For this review, take the finished solid that the model builds, in its own axes (mm). A direction names the side the tool comes from. Give positions to 0.01 mm unless a question says otherwise; leave off trailing zeros. Write each loop counter-clockwise with the first axis right and the second up, starting at its lowest first coordinate (ties: lowest second). Pieces come first, ordered by that corner, then holes. Notation, with made-up numbers: M -12,65.5 L 23,65.5 A23 ccw 23,75.5 Z; hole C 41,-16 d1. An arc over 180 degrees is marked long. Answer as a JSON object with one key per item and string values. Group by question number.
```python
from build123d import *

# Parameters (mm, degrees)
SKETCH_1_R           = 6
EXTRUDE_1_DEPTH      = 6
SKETCH_2_R           = 3
EXTRUDE_2_DEPTH      = 15
SKETCH_4_OUTSIDE_W   = 19.4
SKETCH_4_OUTSIDE_H   = 19.4
CUT_EXTRUDE_1_DEPTH  = 12
SKETCH_5_R           = 18.5
EXTRUDE_3_DEPTH      = 39
EXTRUDE_START        = 6
SKETCH_6_R           = 6
EXTRUDE_4_DEPTH      = 6
SKETCH_7_W           = 38
SKETCH_7_H           = 38
EXTRUDE_5_DEPTH      = 8
EXTRUDE_6_REACH      = 71.176
EXTRUDE_6_END_RADIUS = 18.5
SKETCH_8_W           = 38
SKETCH_8_H           = 26.2
SKETCH_9_R           = 17.9
EXTRUDE_7_DEPTH      = 27
SKETCH_10_R          = 5
EXTRUDE_8_DEPTH      = 2.5
SKETCH_11_R          = 1.5
CUT_EXTRUDE_2_DEPTH  = 4
FILLET_1_R           = 1.5


with BuildPart() as part:
    # Sketch 1 → Extrude 1 (new body)
    with BuildSketch(Plane.XY):
        Circle(SKETCH_1_R)
    extrude(amount=EXTRUDE_1_DEPTH)

    # Sketch 2 → Extrude 2 (add)
    with BuildSketch(Plane.XY.offset(6)):
        Circle(SKETCH_2_R)
    extrude(amount=EXTRUDE_2_DEPTH)

    # Sketch 4 outside → Cut-Extrude 1 (cut)
    with BuildSketch(Plane.XY.offset(21)):
        Rectangle(SKETCH_4_OUTSIDE_W, SKETCH_4_OUTSIDE_H)
        with BuildLine():
            Line((-1.658312395, 2.5), (1.658312395, 2.5))
            ThreePointArc((1.658312395, 2.5), (0, -3), (-1.658312395, 2.5))
        make_face(mode=Mode.SUBTRACT)
    extrude(amount=-CUT_EXTRUDE_1_DEPTH, mode=Mode.SUBTRACT)

    # Sketch 5 → Extrude 3 (add)
    with BuildSketch(Plane.XY):
        with Locations((0, -7)):
            Circle(SKETCH_5_R)
    extrude(amount=-EXTRUDE_3_DEPTH)

    # Sketch 6 → Extrude 4 (add)
    with BuildSketch(Plane(origin=(0, 0, -39), x_dir=(-1, 0, 0), z_dir=(0, 0, -1)).offset(EXTRUDE_START)):
        with Locations(Location((0, 0, 0), (0, 0, 180))):
            Circle(SKETCH_6_R)
    extrude(amount=-EXTRUDE_4_DEPTH)



with BuildPart() as body_2:
    # Sketch 7 → Extrude 5 (new body)
    with BuildSketch(Plane(origin=(26.5, 0, 0), x_dir=(0, 0, -1), z_dir=(1, 0, 0))):
        with Locations((19.5, -18.3)):
            Rectangle(SKETCH_7_W, SKETCH_7_H)
    extrude(amount=-EXTRUDE_5_DEPTH)


with BuildPart() as part_1:
    add(part.part)

    add(body_2.part)  # Extrude 6 merges body 2
    # Extrude 6: up to this cylinder (the profile starts outside it)
    extrude_6_end = Plane(origin=(0, -7, -19.5), z_dir=(0, 0, 1)) * Cylinder(EXTRUDE_6_END_RADIUS, 180.352, mode=Mode.PRIVATE)
    # Sketch 8 → Extrude 6 (add, up to the surface)
    with BuildSketch(Plane.ZY.offset(-18.5), mode=Mode.PRIVATE) as extrude_6_sk1:
        with Locations((-19.5, -12.4)):
            Rectangle(SKETCH_8_W, SKETCH_8_H)
    extrude_6_tool1 = extrude(extrude_6_sk1.sketch, amount=EXTRUDE_6_REACH, mode=Mode.PRIVATE) - extrude_6_end
    add(extrude_6_tool1.solids().sort_by_distance((18.5, -12.4, -19.5))[0])
    add(extrude_6_tool1.solids().sort_by_distance((18.5, -12.4, -19.5))[1])

    # Sketch 9 → Extrude 7 (add)
    with BuildSketch(Plane(origin=(26.5, 0, 0), x_dir=(0, 0, -1), z_dir=(1, 0, 0))):
        with Locations((19.5, -18.3)):
            Circle(SKETCH_9_R)
    extrude(amount=EXTRUDE_7_DEPTH)

    # Sketch 10 → Extrude 8 (add)
    with BuildSketch(Plane(origin=(53.5, 0, 0), x_dir=(0, 0, -1), z_dir=(1, 0, 0))):
        with Locations((19.5, -18.3)):
            Circle(SKETCH_10_R)
    extrude(amount=EXTRUDE_8_DEPTH)

    # Sketch 11 → Cut-Extrude 2 (cut)
    with BuildSketch(Plane.XY):
        with Locations((-15.5, -7)):
            Circle(SKETCH_11_R)
        with Locations((-7.75, 6.423393759)):
            Circle(SKETCH_11_R)
        with Locations((7.75, 6.423393759)):
            Circle(SKETCH_11_R)
        with Locations((15.5, -7)):
            Circle(SKETCH_11_R)
        with Locations((7.75, -20.423393759)):
            Circle(SKETCH_11_R)
        with Locations((-7.75, -20.423393759)):
            Circle(SKETCH_11_R)
    extrude(amount=-CUT_EXTRUDE_2_DEPTH, mode=Mode.SUBTRACT)

    # Fillet 1
    fillet_1_edges = [part_1.edges().sort_by_distance(p)[0] for p in [
        (18.5, -25.5, -19.5),
    ]]
    fillet(fillet_1_edges, radius=FILLET_1_R)


solid = part_1.part
```
Item 1: Consider section D-D (x = -15.5). Give the boundary of the cut face in (y, z).
Item 2: Draft analysis for pull direction Y (two halves, no side actions). For faces 4 (the flat face through (-8, 6, -4)), 5 (the cylindrical face through (54.7, -21.3, -15.5)), 6 (the flat face through (18.5, -32, -19)), state which applies: released by +Y, released by -Y, zero draft, split by the parting line, or undercut.
Item 3: Consider section B-B (x = 15.5). Give the boundary of the cut face in (y, z).
Item 4: To check wall thickness, follow probe 1 along Y at (x, z) = (7, -2); probe 2 along Y at (x, z) = (-7.75, -2.4); probe 3 along Y at (x, z) = (15, -3). State the ranges of each line that lie inside material, in increasing order.
Item 5: Machinability: for faces 1 (the cylindrical face through (5.723, -1.802, -42.042)), 2 (the flat face through (53.5, -22, -23.2)), 3 (the flat face through (-3, -1, 6)), which of the approach directions +Z, -Z, +X, -X, +Y, -Y give a long, thin tool a straight path to every point of the face, cutting with its end or side? Answer none if there is none.
Item 6: Insertion check: P1, Ø11, axis at x = 8.5, y = 2, coming from the +Z side; P2, Ø4, axis at x = -7.75, y = -20.42, coming from the -Z side; P3, Ø3, axis at y = 1.5, z = -27, coming from the -X side. Each pin has a flat end and moves straight along its axis. Give the tip position at first contact, or say it passes through.
Item 7: Consider section A-A (z = -11). Give the boundary of the cut face in (x, y), plus the area to 3 significant figures.
Item 8: Consider section C-C (y = -9.5). Give the boundary of the cut face in (x, z).
Result set:
{
 "1": {"outline": "M -17.1,-39 L 3.1,-39 L 3.1,0 L -5.5,0 L -5.5,-4 L -8.5,-4 L -8.5,0 L -17.1,0 Z"},
 "2": {"face 4": "undercut", "face 5": "split by the parting line", "face 6": "zero draft"},
 "3": {"outline": "M -25.5,-38.5 L -17.1,-38.5 L -17.1,-39 L 3.1,-39 L 3.1,0 L -5.5,0 L -5.5,-4 L -8.5,-4 L -8.5,0 L -17.1,0 L -17.1,-0.5 L -25.5,-0.5 Z"},
 "4": {"probe 1": "y = -25.5 to -21.72, -19.12 to 5.12, 7.72 to 10.12", "probe 2": "y = -23.8 to -21.92, -18.92 to 4.92, 7.92 to 9.8", "probe 3": "y = -25.5 to -8.41, -5.59 to 3.83"},
 "5": {"face 1": "-Z", "face 2": "+X", "face 3": "+Z"},
 "6": {"P1": "stops at z = 6", "P2": "stops at z = -39", "P3": "stops at x = -17.12"},
 "7": {"outline": "M 0,-25.5 L 17,-25.5 A1.5 cw 18.5,-27 L 18.5,-37.3 L 26.5,-37.3 L 26.5,-34.05 L 53.5,-34.05 L 53.5,-2.55 L 26.5,-2.55 L 26.5,0.7 L 16.82,0.7 A18.5 ccw long Z", "area": "2,310 mm^2"},
 "8": {"outline": "M -18.33,-39 L 18.33,-39 L 18.33,-38.5 L 26.5,-38.5 L 26.5,-35.09 L 53.5,-35.09 L 53.5,-3.91 L 26.5,-3.91 L 26.5,-0.5 L 18.33,-0.5 L 18.33,0 L -18.33,0 Z"}
}
